Design review of the part built by this model. Coordinates are the model's own, in mm. Give positions to 0.01 mm unless a question says otherwise; leave off trailing zeros. Write each loop counter-clockwise with the first axis right and the second up, starting at its lowest first coordinate (ties: lowest second). Pieces come first, ordered by that corner, then holes. Notation, with made-up numbers: M 19.5,31 L 28.5,31 A22 cw 28.5,40 Z; hole C -29,-22 d2. An arc over 180 degrees is marked long. Use one line per item in the form item = value. Start each with the question number.
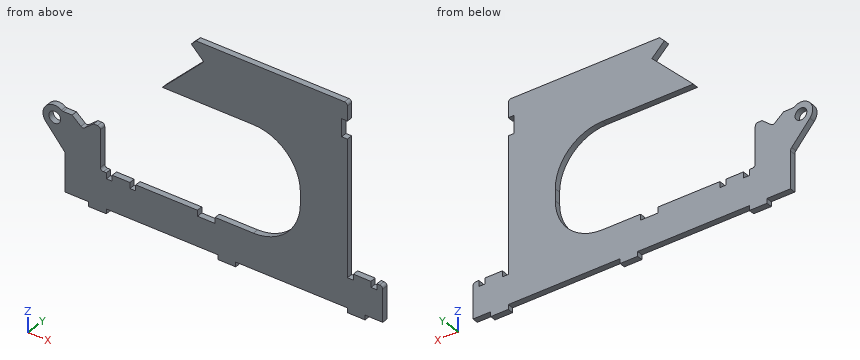
from build123d import *

# Parameters (mm, degrees)
F0_R     = 6.35
F0_W     = 19.05
F0_H     = 5.08
F1_DEPTH = 6.35
F2_R     = 3.175
F3_R     = 5.08
F4_R     = 3.175
F5_R     = 3.175


# Not quite as in the source:
# - ends of sketch curves that miss each other by under 0.0002 mm in the source are joined


with BuildPart() as f1:
    # F0 (on Front) → F1 (new body)
    with BuildSketch(Plane.XZ):
        with BuildLine():
            Line((-72.7094654823, -50.272475262), (-83.3648741359, -50.272475262))
            ThreePointArc((-83.3648741359, -50.272475262), (-100.4842470659, -51.222143603), (-101.056400417, -68.3582903151))
            Line((-101.056400417, -68.3582903151), (-80.147210941, -92.8018072064))
            Line((-80.147210941, -92.8018072064), (-80.147210941, -134.409975262))
            Line((-80.147210941, -134.409975262), (-54.747210941, -134.409975262))
            Line((-54.747210941, -134.409975262), (-35.697210941, -134.409975262))
            Line((-35.697210941, -134.409975262), (84.952789059, -134.409975262))
            Line((84.952789059, -134.409975262), (104.002789059, -134.409975262))
            Line((104.002789059, -134.409975262), (224.652789059, -134.409975262))
            Line((224.652789059, -134.409975262), (243.702789059, -134.409975262))
            Line((243.702789059, -134.409975262), (262.752789059, -134.409975262))
            Line((262.752789059, -134.409975262), (262.752789059, -96.309975262))
            Line((262.752789059, -96.309975262), (256.402789059, -96.309975262))
            Line((256.402789059, -96.309975262), (256.402789059, -102.659975262))
            Line((256.402789059, -102.659975262), (250.052789059, -102.659975262))
            Line((250.052789059, -102.659975262), (250.052789059, -96.309975262))
            Line((250.052789059, -96.309975262), (231.002789059, -96.309975262))
            Line((231.002789059, -96.309975262), (231.002789059, -102.659975262))
            Line((231.002789059, -102.659975262), (224.652789059, -102.659975262))
            Line((224.652789059, -102.659975262), (224.652789059, 43.390024738))
            Line((224.652789059, 43.390024738), (218.302789059, 43.390024738))
            Line((218.302789059, 43.390024738), (218.302789059, 62.440024738))
            Line((218.302789059, 62.440024738), (224.652789059, 62.440024738))
            Line((224.652789059, 62.440024738), (224.652789059, 81.490024738))
            Line((224.652789059, 81.490024738), (61.4126609984, 81.490024738))
            Line((61.4126609984, 81.490024738), (56.0792184251, 76.1565821646))
            Line((56.0792184251, 76.1565821646), (69.5496026067, 62.686197983))
            Line((69.5496026067, 62.686197983), (24.8534293616, 17.990024738))
            Line((24.8534293616, 17.990024738), (123.052789059, 17.990024738))
            ThreePointArc((123.052789059, 17.990024738), (158.9738135432, 3.1110492223), (173.852789059, -32.809975262))
            Line((173.852789059, -32.809975262), (173.852789059, -45.509975262))
            ThreePointArc((173.852789059, -45.509975262), (158.9738135432, -81.4309997463), (123.052789059, -96.309975262))
            Line((123.052789059, -96.309975262), (81.777789059, -96.309975262))
            Line((81.777789059, -96.309975262), (81.777789059, -102.659975262))
            Line((81.777789059, -102.659975262), (62.727789059, -102.659975262))
            Line((62.727789059, -102.659975262), (62.727789059, -96.309975262))
            Line((62.727789059, -96.309975262), (-3.947210941, -96.309975262))
            Line((-3.947210941, -96.309975262), (-3.947210941, -102.659975262))
            Line((-3.947210941, -102.659975262), (-10.297210941, -102.659975262))
            Line((-10.297210941, -102.659975262), (-10.297210941, -96.309975262))
            Line((-10.297210941, -96.309975262), (-29.347210941, -96.309975262))
            Line((-29.347210941, -96.309975262), (-29.347210941, -102.659975262))
            Line((-29.347210941, -102.659975262), (-35.697210941, -102.659975262))
            Line((-35.697210941, -102.659975262), (-35.697210941, -96.309975262))
            Line((-35.697210941, -96.309975262), (-42.047210941, -96.309975262))
            Line((-42.047210941, -96.309975262), (-42.047210941, -50.272475262))
            Line((-42.047210941, -50.272475262), (-49.4849563998, -50.272475262))
            Line((-49.4849563998, -50.272475262), (-61.097210941, -60.0163137647))
            Line((-61.097210941, -60.0163137647), (-72.7094654823, -50.272475262))
        make_face()
        with Locations((-91.4055753496, -60.1028935639)):
            Circle(F0_R, mode=Mode.SUBTRACT)
        with Locations((-45.222210941, -136.949975262)):
            Rectangle(F0_W, F0_H)
        with Locations((94.477789059, -136.949975262)):
            Rectangle(F0_W, F0_H)
        with Locations((234.177789059, -136.949975262)):
            Rectangle(F0_W, F0_H)
    extrude(amount=-F1_DEPTH)

    # F2
    f2_edges = [f1.edges().sort_by_distance(p)[0] for p in [
        (224.652789, 3.175, 81.490025),
        (-42.047211, 3.175, -96.309975),
    ]]
    fillet(f2_edges, radius=F2_R)

    # F3
    f3_edges = [f1.edges().sort_by_distance(p)[0] for p in [
        (-80.147211, 3.175, -92.801807),
    ]]
    fillet(f3_edges, radius=F3_R)

    # F4
    f4_edges = [f1.edges().sort_by_distance(p)[0] for p in [
        (-42.047211, 3.175, -50.272475),
    ]]
    fillet(f4_edges, radius=F4_R)

    # F5
    f5_edges = [f1.edges().sort_by_distance(p)[0] for p in [
        (-61.097211, 3.175, -60.016314),
        (-83.364874, 3.175, -50.272475),
        (262.752789, 3.175, -96.309975),
    ]]
    fillet(f5_edges, radius=F5_R)


solid = f1.part
1. We need section C-C (x = 17.5). State the section outline as (y, z) points.
2. To check wall thickness, follow L1, parallel to Z at x = 86.5, y = 5; L2, parallel to X at y = 0.75, z = -55.5; L3, parallel to Z at x = 124.5, y = 1.5. State the ranges of each line that lie inside material, in increasing order.
3. We need section D-D (z = -42). State the section outline as (x, y) points.
4. Clearance check with flat-ended pins moving along their axes: pin 1 Ø3 at (x, y) = (-16.5, 2) entering from +Z; pin 2 Ø1.5 at (x, y) = (68.5, 0.5) entering from -Z; pin 3 Ø1.9 at (x, y) = (-32, 2) entering from +Z. State where each tip first meets the part, or that it passes through.
5. We need section A-A (x = 90.5). State the section outline as (y, z) points.
6. We need section B-B (z = -74.5). State the section outline as (x, y) points.
Answer block:
q1.outline = M 0,-134.41 L 6.35,-134.41 L 6.35,-96.31 L 0,-96.31 Z
q2.L1 = -139.49 to -96.31, 17.99 to 81.49
q2.L2 = -103.24 to -95.78, -87.03 to -66.48, -55.71 to -42.05, 172.86 to 224.65
q2.L3 = -134.41 to -96.29, 17.97 to 81.49
q3.outline = M 173.85,0 L 224.65,0 L 224.65,6.35 L 173.85,6.35 Z
q4.pin_1 = -96.31
q4.pin_2 = -134.41
q4.pin_3 = -102.66
q5.outline = M 0,-139.49 L 6.35,-139.49 L 6.35,-96.31 L 0,-96.31 Z; M 0,17.99 L 6.35,17.99 L 6.35,81.49 L 0,81.49 Z
q6.outline = M -95.8,0 L -42.05,0 L -42.05,6.35 L -95.8,6.35 Z; M 164.77,0 L 224.65,0 L 224.65,6.35 L 164.77,6.35 Z
